Geometry check sheet. Reference: the model listing, model coordinates, mm. Face numbers are marked on the shaded views. Round coordinates to 2 decimals unless told otherwise and drop trailing zeros. Loops run counter-clockwise (first coordinate to the right, second up) from the corner with the lowest first, then second, coordinate; pieces in that order, holes last. Notation, with made-up numbers: (21.5, 66.25) - (73.5, 66.25) arc R17 ccw to (73.5, 91.25) - close; hole circle Ø2 at (29.25, 77.25). An arc over 180 degrees is marked (long way). Write item = value, one per line.
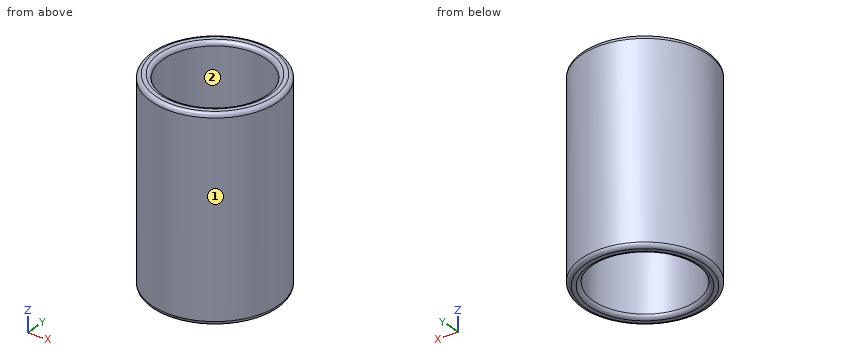
```python
from build123d import *

# Parameters (mm, degrees)
CYLINDER001_R     = 13
CYLINDER001_DEPTH = 120
CYLINDER_R        = 16
CYLINDER_DEPTH    = 50
FILLET_R          = 1


with BuildPart() as obj1:
    # Cylinder001 → Cylinder001 (new body)
    with BuildSketch(Plane.XY.offset(-60)):
        Circle(CYLINDER001_R)
    extrude(amount=CYLINDER001_DEPTH)


with BuildPart() as fillet_body:
    # Cylinder → Cylinder (new body)
    with BuildSketch(Plane.XY.offset(-60)):
        Circle(CYLINDER_R)
    extrude(amount=CYLINDER_DEPTH)

    # Cut: cut obj1
    add(obj1.part, mode=Mode.SUBTRACT)

    # Fillet
    fillet_edges = [fillet_body.edges().sort_by_distance(p)[0] for p in [
        (-16, 0, -10),
        (-16, 0, -60),
        (-13, 0, -10),
        (-13, 0, -60),
    ]]
    fillet(fillet_edges, radius=FILLET_R)


solid = fillet_body.part
```
(1) Scan lines: L1, parallel to Y at x = 0.5, z = -41.5; L2, parallel to Y at x = 3, z = -36; L3, parallel to X at y = 7.5, z = -34.5. Record each from-to range of solid material in increasing order. Write a range as [from, to].
Answers follow:
L1 = [-15.99, -12.99], [12.99, 15.99]
L2 = [-15.72, -12.65], [12.65, 15.72]
L3 = [-14.13, -10.62], [10.62, 14.13]
(2) Gauge pin test, flat ends, axial feed: pin 1 (4 mm diameter, centred on x = 3.5, y = -9.5, fed in from -Z); pin 2 (5 mm diameter, centred on y = 7.5, z = -54, fed in from -X); pin 3 (4 mm diameter, centred on x = 10.5, z = -36, fed in from +Y); pin 4 (10 mm diameter, centred on y = -8.5, z = -38, fed in from -X). Record the tip position at first contact, or that the pin passes through.
Answers follow:
pin_1 = through
pin_2 = -15.2
pin_3 = 13.56
pin_4 = -15.61
(3) Mould release check, pull along X, two halves, no side actions. Record for the marked faces 1 and 2: pulls with the +X half, pulls with the -X half, needs draft (parallel to the pull), parting line crosses it, or undercut.
Answers follow:
face_1 = parting line crosses it
face_2 = undercut
(4) Section check A-A (y = 0). Enter the section's corners in (x, z).
Answers follow:
outline = (-16, -59) arc R1 ccw to (-15, -60) - (-14, -60) arc R1 ccw to (-13, -59) - (-13, -11) arc R1 ccw to (-14, -10) - (-15, -10) arc R1 ccw to (-16, -11) - close; (13, -59) arc R1 ccw to (14, -60) - (15, -60) arc R1 ccw to (16, -59) - (16, -11) arc R1 ccw to (15, -10) - (14, -10) arc R1 ccw to (13, -11) - close
(5) Section check C-C (z = -25.5). Enter the section's corners in (x, y), then the cut area to 3 significant figures.
Answers follow:
outline = circle Ø32 at (0, 0); hole circle Ø26 at (0, 0)
area = 273 mm²
